Source: CAD feature listing. Evaluate the final solid. Frame: model axes, mm. A direction names the side the tool comes from. Round coordinates to 2 decimals unless told otherwise and drop trailing zeros. Order: outer loops, then holes, each group sorted by start corner. A loop starts at its lowest first (then second) coordinate and runs counter-clockwise, first axis right, second up. Notation, with made-up numbers: (-17.75, 61.25) -> (24.25, 61.25) arc R30 ccw to (24.25, 83.25) -> close; hole circle Ø9 at (83.5, 38.5). An arc over 180 degrees is marked (long way). One line per item, written item: value. Start each with the question number.
1) Pin query (flat end, axial travel): P1, Ø6, axis at x = 14, z = -3.5, coming from the +Y side. Return the tip coordinate at first contact, or that it passes through.
2) Mould query, pull axis X, two halves, no side actions, for faces 1 (the face through (19, -33, -4)), 2 (the face through (6, -28, -4)), 3 (the face through (30, -26, -4)). Classes: pulls with the +X half, pulls with the -X half, needs draft (parallel to the pull), parting line crosses it, or undercut.
3) Section D-D (y = -31.75). Return the cut outline in (x, z).
4) Reachability of faces 4 (the face through (18.32, -31.48, 0.58)), 5 (the face through (9, -26, -4)) from +Z, -Z, +X, -X, +Y, -Y: full face, straight path, thin tool, end or side. Return the list, or none.
5) Section B-B (y = -28.5). Return the cut outline in (x, z), and give its area (3 significant figures).
6) Section C-C (x = 19.5). Return the cut outline in (y, z), and give its area (3 significant figures).
7) Ray query, L1, parallel to X at y = -25.5, z = 1.75; L2, parallel to Z at x = 19.5, y = -31.6; L3, parallel to Y at x = 16, z = -5.5. Return the intervals inside material, ascending.
8) Section A-A (z = -8.5). Return the cut outline in (x, y), and give its area (3 significant figures).
```python
from build123d import *

# Parameters (mm, degrees)
CYLINDER976_R          = 1.6
CYLINDER976_DEPTH      = 20
CYLINDER976_ROLL_ANGLE = 90
CYLINDER975_R          = 1.6
CYLINDER975_DEPTH      = 20
CYLINDER975_ROLL_ANGLE = 90
BOX493_W               = 16
BOX493_H               = 10
BOX493_DEPTH           = 3
BOX492_W               = 16
BOX492_H               = 10
BOX492_DEPTH           = 3
BOX491_W               = 16
BOX491_H               = 3
BOX491_DEPTH           = 21
FUSION493_PITCH_ANGLE  = 90


with BuildPart() as cylinder1038:
    # Cylinder976 → Cylinder976 (new body)
    with BuildSketch(Plane.XY):
        Circle(CYLINDER976_R)
    extrude(amount=CYLINDER976_DEPTH)


with BuildPart() as cylinder1038_1:
    # Cylinder976 roll: moved
    add(cylinder1038.part.rotate(Axis((0, 0, 0), (1, 0, 0)), CYLINDER976_ROLL_ANGLE))


with BuildPart() as cylinder1038_2:
    # Cylinder976 placement: moved
    add(cylinder1038_1.part.moved(Location((19.5, 30, 0.5))))


with BuildPart() as fusion112:
    # Cylinder975 → Cylinder975 (new body)
    with BuildSketch(Plane.XY):
        Circle(CYLINDER975_R)
    extrude(amount=CYLINDER975_DEPTH)


with BuildPart() as fusion112_1:
    # Cylinder975 roll: moved
    add(fusion112.part.rotate(Axis((0, 0, 0), (1, 0, 0)), CYLINDER975_ROLL_ANGLE))


with BuildPart() as fusion112_2:
    # Cylinder975 placement: moved
    add(fusion112_1.part.moved(Location((19.5, 30, -7.5))))

    # Fusion112: union Cylinder1038
    add(cylinder1038_2.part)


with BuildPart() as fusion112_3:
    # Fusion112 placement: moved
    add(fusion112_2.part.moved(Location((0, -43, -1))))


with BuildPart() as cube695:
    # Box493 → Box493 (new body)
    with BuildSketch(Plane(origin=(128, 50.5, -0.5), x_dir=(1, 0, 0), z_dir=(0, 0, 1))):
        with Locations((8, 5)):
            Rectangle(BOX493_W, BOX493_H)
    extrude(amount=BOX493_DEPTH)


with BuildPart() as cube694:
    # Box492 → Box492 (new body)
    with BuildSketch(Plane(origin=(128, 50.5, -24.5), x_dir=(1, 0, 0), z_dir=(0, 0, 1))):
        with Locations((8, 5)):
            Rectangle(BOX492_W, BOX492_H)
    extrude(amount=BOX492_DEPTH)


with BuildPart() as diff_box_mount_holes:
    # Box491 → Box491 (new body)
    with BuildSketch(Plane(origin=(128, 50.5, -21.5), x_dir=(1, 0, 0), z_dir=(0, 0, 1))):
        with Locations((8, 1.5)):
            Rectangle(BOX491_W, BOX491_H)
    extrude(amount=BOX491_DEPTH)

    # Fusion493: union Cube695, Cube694
    add(cube695.part)
    add(cube694.part)


with BuildPart() as diff_box_mount_holes_1:
    # Fusion493 pitch: moved
    add(diff_box_mount_holes.part.rotate(Axis((0, 0, 0), (0, 1, 0)), FUSION493_PITCH_ANGLE))


with BuildPart() as diff_box_mount_holes_2:
    # Fusion493 placement: moved
    add(diff_box_mount_holes_1.part.moved(Location((30.5, -83.5, 131.5))))

    # Cut014057: cut Fusion112
    add(fusion112_3.part, mode=Mode.SUBTRACT)


solid = diff_box_mount_holes_2.part
```
Findings:
1. P1: y = -30
2. face 1: needs draft
2. face 2: pulls with the -X half
2. face 3: undercut
3. outline: (6, -12.5) -> (33, -12.5) -> (33, 3.5) -> (6, 3.5) -> close; hole circle Ø3.2 at (19.5, -8.5); hole circle Ø3.2 at (19.5, -0.5)
4. face 4: +Y, -Y
4. face 5: +Z, -Z, +Y
5. outline: (6, -12.5) -> (9, -12.5) -> (9, 3.5) -> (6, 3.5) -> close; (30, -12.5) -> (33, -12.5) -> (33, 3.5) -> (30, 3.5) -> close
5. area: 96.0 mm2
6. outline: (-33, -12.5) -> (-30, -12.5) -> (-30, -10.1) -> (-33, -10.1) -> close; (-33, -6.9) -> (-30, -6.9) -> (-30, -2.1) -> (-33, -2.1) -> close; (-33, 1.1) -> (-30, 1.1) -> (-30, 3.5) -> (-33, 3.5) -> close
6. area: 28.8 mm2
7. L1: 6 to 9, 30 to 33
7. L2: -12.5 to -10.1, -6.9 to -2.1, 1.1 to 3.5
7. L3: -33 to -30
8. outline: (6, -33) -> (17.9, -33) -> (17.9, -30) -> (9, -30) -> (9, -23) -> (6, -23) -> close; (21.1, -33) -> (33, -33) -> (33, -23) -> (30, -23) -> (30, -30) -> (21.1, -30) -> close
8. area: 113 mm2
